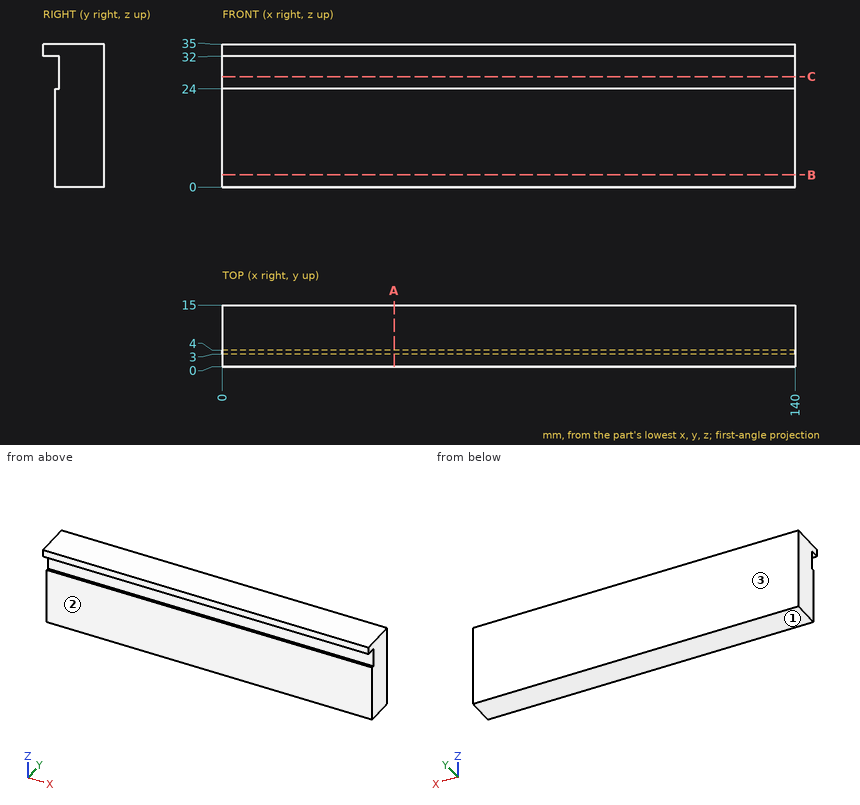
For this review, use the dimensioned drawing (mm, ordinates from the lowest corner) and the shaded views. Coordinates: 2 decimals unless noted, no trailing zeros. Loops run counter-clockwise (first coordinate to the right, second up) from the corner with the lowest first, then second, coordinate; pieces in that order, holes last. Notation, with made-up numbers: (22.5, 37) -> (71.5, 37) arc R28 cw to (71.5, 73) -> close; hole circle Ø2 at (30.25, 50.25). An arc over 180 degrees is marked (long way). Use a Markdown table: item, result. Add a question column.
1. Add section A-A on x = 42. Write out the cut boundary in (y, z).
2. To check wall thickness, follow line 1 (Z direction, x = 85, y = 3.5); line 2 (Y direction, x = 114.5, z = 20); line 3 (Y direction, x = 123, z = 24.5). State the ranges of each line that lie inside material, in increasing order.
3. Add section C-C on z = 27. Write out the cut boundary in (x, y).
4. Clearance check with flat-ended pins moving along their axes: pin 1 Ø4 at (x, z) = (105, 14) entering from -Y; pin 2 Ø2.5 at (x, z) = (77.5, 27.5) entering from -Y. State where each tip first meets the part, or that it passes through.
5. Add section B-B on z = 3. Write out the cut boundary in (x, y), plus the area to 3 significant figures.
6. Draft analysis for pull direction Y (two halves, no side actions). For the marked faces 1, 2 and 3, state which applies: pulls with the +Y half, pulls with the -Y half, needs draft (parallel to the pull), parting line crosses it, or undercut.
Returned:
| question | item | result |
|---|---|---|
| 1 | outline | (0, 32) -> (4, 32) -> (4, 24) -> (3, 24) -> (3, 0) -> (15, 0) -> (15, 35) -> (0, 35) -> close |
| 2 | line 1 | z = 0 to 24, 32 to 35 |
| 2 | line 2 | y = 3 to 15 |
| 2 | line 3 | y = 4 to 15 |
| 3 | outline | (0, 4) -> (140, 4) -> (140, 15) -> (0, 15) -> close |
| 4 | pin 1 | stops at y = 3 |
| 4 | pin 2 | stops at y = 4 |
| 5 | outline | (0, 3) -> (140, 3) -> (140, 15) -> (0, 15) -> close |
| 5 | area | 1,680 mm² |
| 6 | face 1 | needs draft |
| 6 | face 2 | pulls with the -Y half |
| 6 | face 3 | pulls with the +Y half |
